Design review of the part built by this model. Coordinates are the model's own, in mm. Coordinates: 2 decimals unless noted, no trailing zeros. Loops run counter-clockwise (first coordinate to the right, second up) from the corner with the lowest first, then second, coordinate; pieces in that order, holes last. Notation, with made-up numbers: (-28, -25.75) -> (-6, -25.75) arc R26 cw to (-6, 12.25) -> close; hole circle Ø7 at (27, 28.5). An arc over 180 degrees is marked (long way). Use CSV: the item, a comma, the result in double quotes.
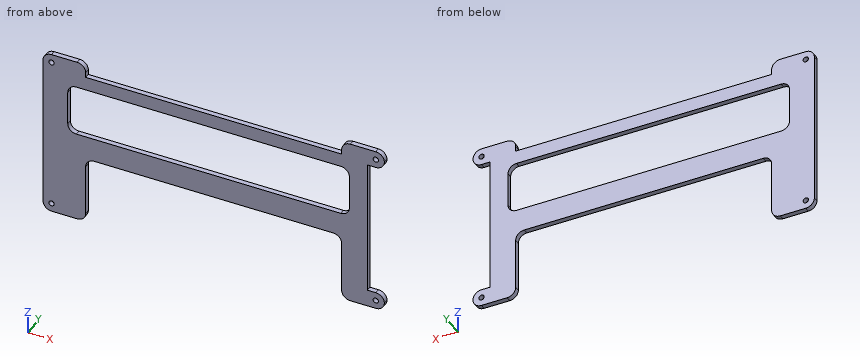
```python
from build123d import *

# Parameters (mm, degrees)
SKETCH1_W           = 200
SKETCH1_H           = 100
BOSS_EXTRUDE1_DEPTH = 3
SKETCH2_R           = 1.55
CUT_EXTRUDE1_DEPTH  = 112.843640856
FILLET1_R           = 5
SKETCH3_W           = 150
SKETCH3_H           = 40
SKETCH3_W_2         = 10
SKETCH3_H_2         = 80
SKETCH3_H_3         = 8
SKETCH3_W_3         = 165
SKETCH3_H_4         = 30
CUT_EXTRUDE2_DEPTH  = 112.843640856
FILLET2_START       = -1
FILLET2_DEPTH       = 5
FILLET2_2_DEPTH     = 3


with BuildPart() as part:
    # Sketch1 → Boss-Extrude1 (new body)
    with BuildSketch(Plane(origin=(0, 0, 0), x_dir=(1, 0, 0), z_dir=(0, 1, 0))):
        Rectangle(SKETCH1_W, SKETCH1_H)
    extrude(amount=BOSS_EXTRUDE1_DEPTH)

    # Sketch2 → Cut-Extrude1 (cut, through all)
    with BuildSketch(Plane(origin=(0, 3, 0), x_dir=(1, 0, 0), z_dir=(0, 1, 0))):
        with Locations(Location((-95, 45, 0), (0, 0, 270))):
            Circle(SKETCH2_R)
        with Locations(Location((-95, -45, 0), (0, 0, 270))):
            Circle(SKETCH2_R)
        with Locations(Location((95, 45, 0), (0, 0, 270))):
            Circle(SKETCH2_R)
        with Locations(Location((95, -45, 0), (0, 0, 270))):
            Circle(SKETCH2_R)
    extrude(amount=-CUT_EXTRUDE1_DEPTH, mode=Mode.SUBTRACT)

    # Fillet1
    fillet1_edges = [part.edges().sort_by_distance(p)[0] for p in [
        (-100, 1.5, -50),
        (100, 1.5, -50),
        (100, 1.5, 50),
        (-100, 1.5, 50),
    ]]
    fillet(fillet1_edges, radius=FILLET1_R)

    # Sketch3 → Cut-Extrude2 (cut, through all)
    with BuildSketch(Plane(origin=(0, 3, 0), x_dir=(1, 0, 0), z_dir=(0, 1, 0))):
        with Locations((0, 30)):
            Rectangle(SKETCH3_W, SKETCH3_H)
        with Locations((95, 0)):
            Rectangle(SKETCH3_W_2, SKETCH3_H_2)
        with Locations((0, -46)):
            Rectangle(SKETCH3_W, SKETCH3_H_3)
        with Locations((-3, -19)):
            Rectangle(SKETCH3_W_3, SKETCH3_H_4)
    extrude(amount=-CUT_EXTRUDE2_DEPTH, mode=Mode.SUBTRACT)

    # Fillet2: read off the stored shape, not the designer's step
    # Fillet2 outline → Fillet2 (cut)
    with BuildSketch(Plane(origin=(0, 0, 0), x_dir=(1, 0, 0), z_dir=(0, 1, 0)).offset(FILLET2_START)):
        with BuildLine():
            Line((100, 40), (100, 45))
            ThreePointArc((100, 45), (98.535533906, 41.464466094), (95, 40))
            Line((95, 40), (100, 40))
        make_face()
        with BuildLine():
            ThreePointArc((-80, 50), (-76.464466094, 48.535533906), (-75, 45))
            Line((-75, 45), (-75, 50))
            Line((-75, 50), (-80, 50))
        make_face()
        with BuildLine():
            ThreePointArc((75, 45), (76.464466094, 48.535533906), (80, 50))
            Line((80, 50), (75, 50))
            Line((75, 50), (75, 45))
        make_face()
        with BuildLine():
            Line((100, -40), (95, -40))
            ThreePointArc((95, -40), (98.535533906, -41.464466094), (100, -45))
            Line((100, -45), (100, -40))
        make_face()
        with BuildLine():
            Line((75, -50), (80, -50))
            ThreePointArc((80, -50), (76.464466094, -48.535533906), (75, -45))
            Line((75, -45), (75, -50))
        make_face()
        with BuildLine():
            ThreePointArc((-75, -45), (-76.464466094, -48.535533906), (-80, -50))
            Line((-80, -50), (-75, -50))
            Line((-75, -50), (-75, -45))
        make_face()
    extrude(amount=FILLET2_DEPTH, mode=Mode.SUBTRACT)

    # Fillet2 2 outline → Fillet2 2 (add)
    with BuildSketch(Plane(origin=(0, 0, 0), x_dir=(1, 0, 0), z_dir=(0, 1, 0))):
        with BuildLine():
            Line((-75, 10), (-70, 10))
            ThreePointArc((-70, 10), (-73.535533906, 11.464466094), (-75, 15))
            Line((-75, 15), (-75, 10))
        make_face()
        with BuildLine():
            Line((75, 10), (75, 15))
            ThreePointArc((75, 15), (73.535533906, 11.464466094), (70, 10))
            Line((70, 10), (75, 10))
        make_face()
        with BuildLine():
            Line((79.5, -34), (79.5, -29))
            ThreePointArc((79.5, -29), (78.035533906, -32.535533906), (74.5, -34))
            Line((74.5, -34), (79.5, -34))
        make_face()
        with BuildLine():
            ThreePointArc((74.5, -4), (78.035533906, -5.464466094), (79.5, -9))
            Line((79.5, -9), (79.5, -4))
            Line((79.5, -4), (74.5, -4))
        make_face()
        with BuildLine():
            Line((-85.5, -34), (-80.5, -34))
            ThreePointArc((-80.5, -34), (-84.035533906, -32.535533906), (-85.5, -29))
            Line((-85.5, -29), (-85.5, -34))
        make_face()
        with BuildLine():
            ThreePointArc((-85.5, -9), (-84.035533906, -5.464466094), (-80.5, -4))
            Line((-80.5, -4), (-85.5, -4))
            Line((-85.5, -4), (-85.5, -9))
        make_face()
    extrude(amount=FILLET2_2_DEPTH)


solid = part.part
```
Item 1: Clearance check with flat-ended pins moving along their axes: pin 1 (1.5 mm diameter, centred on x = 11.5, y = 2, fed in from -Z); pin 2 (1.5 mm diameter, centred on x = 13.5, y = 2, fed in from +Z); pin 3 (5 mm diameter, centred on x = -95, z = -45, fed in from +Y); pin 4 (1.9 mm diameter, centred on x = -95, z = 45, fed in from +Y). State where each tip first meets the part, or that it passes through.
Checked values:
pin 1,"z = -10"
pin 2,"z = 42"
pin 3,"y = 3"
pin 4,"through"
Item 2: Add section B-B (x = 3). Give the boundary of the cut face in (y, z).
Checked values:
outline,"(0, -10) -> (3, -10) -> (3, 4) -> (0, 4) -> close; (0, 34) -> (3, 34) -> (3, 42) -> (0, 42) -> close"
Item 3: To check wall thickness, follow line 1 along X through (y, z) = (1.2, -45); line 2 along Z through (x, y) = (-95, 0.95); line 3 along X through (y, z) = (1.4, -30). State the ranges of each line that lie inside material, in increasing order.
Checked values:
line 1,"-100 to -96.55, -93.45 to -75, 75 to 93.45, 96.55 to 100"
line 2,"-50 to -46.55, -43.45 to 43.45, 46.55 to 50"
line 3,"-100 to -75, 75 to 90"
Item 4: Add section A-A (z = 13.5). Give the boundary of the cut face in (x, y), then the cut area to 3 significant figures.
Checked values:
outline,"(-100, 0) -> (-85.5, 0) -> (-85.5, 3) -> (-100, 3) -> close; (79.5, 0) -> (90, 0) -> (90, 3) -> (79.5, 3) -> close"
area,"75.0 mm^2"
Item 5: Add section C-C (y = 2.5). State how many separate pieces and enclosed holes the cut face has, then the cut area to 3 significant figures.
Checked values:
separate pieces,"1"
enclosed holes,"5"
area,"7,000 mm^2"
